Can you work these out from the model? Positions are in its coordinate system, mm. Round coordinates to 2 decimals unless told otherwise and drop trailing zeros. Loops run counter-clockwise (first coordinate to the right, second up) from the corner with the lowest first, then second, coordinate; pieces in that order, holes last.
from build123d import *

# Parameters (mm, degrees)
F2_DEPTH = 1.651
F3_DEPTH = 0.7112
F4_DEPTH = 16.68526
F5_DEPTH = 2.1082


with BuildPart() as f2:
    # F1 (on Right) → F2 (new body)
    with BuildSketch(Plane.YZ):
        with BuildLine():
            Line((-0.2421069604, 13.3002023897), (-0.6375133526, 13.2774123922))
            Line((-0.6375133526, 13.2774123922), (0.6271508173, -8.6645074189))
            ThreePointArc((0.6271508173, -8.6645074189), (1.1764445867, -9.2804609215), (1.9562288653, -9.5507549122))
            Line((1.9562288653, -9.5507549122), (10.3850932792, -9.5507549122))
            Line((10.3850932792, -9.5507549122), (10.3850932792, -9.1546922922))
            Line((10.3850932792, -9.1546922922), (1.9730122271, -9.1546922922))
            ThreePointArc((1.9730122271, -9.1546922922), (1.4228217611, -8.9682207065), (1.0173951252, -8.552155274))
            Line((1.0173951252, -8.552155274), (-0.2421069604, 13.3002023897))
        make_face()
    extrude(amount=-F2_DEPTH)

    # F0 (on Top) → F3 (join)
    with BuildSketch(Plane.XY):
        with BuildLine():
            ThreePointArc((0, 9.231187034), (-1.7012077985, 13.3382659736), (-5.808286738, 15.039473772))
            Line((-5.808286738, 15.039473772), (-13.2799016967, 15.039473772))
            ThreePointArc((-13.2799016967, 15.039473772), (-16.8636996774, 13.5550160436), (-18.3481574059, 9.9712180629))
            Line((-18.3481574059, 9.9712180629), (-18.3481574059, 0))
            Line((-18.3481574059, 0), (-16.9112477452, 0))
            Line((-16.9112477452, 0), (-16.9112477452, 9.9712180629))
            ThreePointArc((-16.9112477452, 9.9712180629), (-15.8476511124, 12.5389674786), (-13.2799016967, 13.6025641114))
            Line((-13.2799016967, 13.6025641114), (-5.808286738, 13.6025641114))
            ThreePointArc((-5.808286738, 13.6025641114), (-2.7172563635, 12.3222174085), (-1.4369096607, 9.231187034))
            Line((-1.4369096607, 9.231187034), (-1.4369096607, 0))
            Line((-1.4369096607, 0), (0, 0))
            Line((0, 0), (0, 9.231187034))
        make_face()
    extrude(amount=F3_DEPTH)

    # F4 (add): a face of the model
    f4_faces = [f2.faces().sort_by_distance(p)[0] for p in [
        (-1.651, -0.4252115949, 13.0355223881),
    ]]
    extrude(f4_faces, amount=F4_DEPTH)

    # F5 (add): a face of the model
    f5_faces = [f2.faces().sort_by_distance(p)[0] for p in [
        (-9.16813, 10.3850932792, -9.3527236022),
    ]]
    extrude(f5_faces, amount=F5_DEPTH)


solid = f2.part
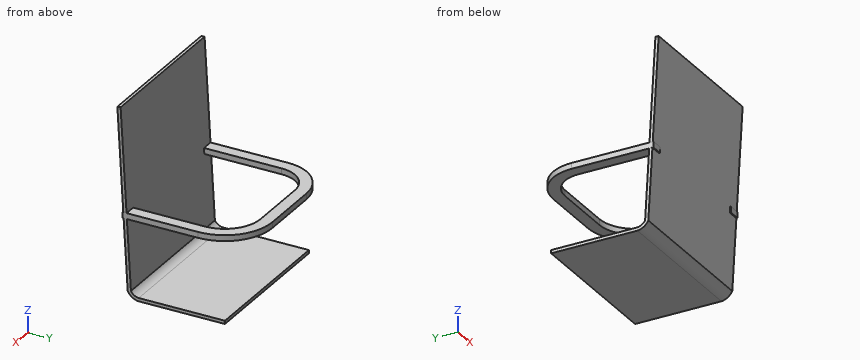
(1) If we section it at B-B, the plane y = 6.5: List the corners of the cut face in (x, z) for me.
Worked answers:
outline: (-18.35, 0) - (-16.91, 0) - (-16.91, 0.71) - (-18.35, 0.71) - close; (-18.34, -9.55) - (0, -9.55) - (0, -9.15) - (-18.34, -9.15) - close; (-1.44, 0) - (0, 0) - (0, 0.71) - (-1.44, 0.71) - close
(2) Will these pins go through, and if not, where does the flat tip stop? P1, Ø0.8, axis at x = -17.5, z = 0.5, coming from the -Y side; P2, Ø0.9, axis at y = 0, z = 9, coming from the -X side; P3, Ø3, axis at x = -14.5, y = 4.5, coming from the +Z side.
Worked answers:
P1: stops at y = 0
P2: stops at x = -18.34
P3: stops at z = -9.15
(3) If we section it at C-C, the plane y = 13.25: List the corners of the cut face in (x, z) for me, then the cut area to 3 significant figures.
Worked answers:
outline: (-17.14, 0) - (-14.84, 0) - (-14.84, 0.71) - (-17.14, 0.71) - close; (-4.09, 0) - (-1.61, 0) - (-1.61, 0.71) - (-4.09, 0.71) - close
area: 3.40 mm2
(4) If we section it at D-D, the plane x = -15.75: List the corners of the cut face in (y, z) for me, then the cut area to 3 significant figures.
Worked answers:
outline: (-0.64, 13.28) - (0.63, -8.66) arc R1.64 ccw to (1.96, -9.55) - (12.49, -9.55) - (12.49, -9.15) - (1.97, -9.15) arc R1.24 cw to (1.02, -8.55) - (-0.24, 13.3) - close; (12.63, 0) - (14.4, 0) - (14.4, 0.71) - (12.63, 0.71) - close
area: 14.7 mm2
(5) If we section it at A-A, the plane x = -7: List the corners of the cut face in (y, z) for me.
Worked answers:
outline: (-0.64, 13.28) - (0.63, -8.66) arc R1.64 ccw to (1.96, -9.55) - (12.49, -9.55) - (12.49, -9.15) - (1.97, -9.15) arc R1.24 cw to (1.02, -8.55) - (-0.24, 13.3) - close; (13.6, 0) - (15.04, 0) - (15.04, 0.71) - (13.6, 0.71) - close
(6) If I drill on line 1 (Z direction, x = -0.75, y = 10.75); line 2 (Z direction, x = -8.5, y = 6.75); line 3 (Y direction, x = -5, z = 0.25), over which ranges is the centre line in solid material (lowest first)?
Worked answers:
line 1: z = -9.55 to -9.15, 0 to 0.71
line 2: z = -9.55 to -9.15
line 3: y = 0.11 to 0.51, 13.53 to 14.98
